Autodesk Inventor part; units mm, degrees
ref_plane "YZ Plane" through (0, 0, 0) normal (1, 0, 0) x (0, 1, 0)
ref_plane "XZ Plane" through (0, 0, 0) normal (0, 1, 0) x (-1, 0, 0)
ref_plane "XY Plane" through (0, 0, 0) normal (0, 0, 1) x (1, 0, 0)
sketch "Sketch1" plane through (0, 0, 0) normal (0, 1, 0) x (-1, 0, 0)
  arc A0 (1.1623, -30.2706) -> (1.1135, 10.0138) centre (15.9463, -10.1104) ccw
  circle A1 centre (15.9463, -10.1104) radius 19
  line L0 (-9.0537, -10.1104) -> (-6.0537, -10.1104)
  line L1 (-6.0537, -10.1104) -> (-6.0537, 49.8896)
  line L2 (-6.0537, 49.8896) -> (-16.0537, 49.8896)
  line L3 (-16.0537, 49.8896) -> (-16.0537, -70.1104)
  line L4 (-16.0537, -70.1104) -> (-6.0537, -70.1104)
  line L5 (-6.0537, -70.1104) -> (-6.0537, -10.1104)
  line L6 (-6.0537, 19.8896) -> (1.1135, 10.0138)
  line L7 (15.9463, -10.1104) -> (15.8318, -10.2667)
  line L8 (1.1623, -30.2706) -> (-6.0537, -40.1104)
  point P0 (0, 0)
  dimension "d0" = 50
  dimension "d1" = 38
  dimension "d2" = 3
  dimension "d4" = 10
  dimension "d5" = 120
  dimension "d11" = 0
extrude "Extrusion1" add sketch "Sketch1" along normal blind 40
sketch "Sketch2" plane through (16.0537, 0, 49.8896) normal (1, 0, 0) x (0, 0, -1)
  line L0 (0, 0) -> (0, 40)
  line L1 (0, 20) -> (120, 20)
  line L2 (120, 0) -> (120, 40)
  circle A0 centre (60, 20) radius 5
  circle A1 centre (20, 20) radius 4
  circle A2 centre (100, 20) radius 4
  point P0 (49.8896, 0)
  dimension "d14" = 10
  dimension "d15" = 8
  dimension "d16" = 8
  dimension "d17" = 20
  dimension "d18" = 20
hole "Hole1" at (16.0537, 20, 29.8896) at (16.0537, 20, -50.1104) direction (-1, 0, 0) diameter 8.376 depth 27.3 tip angle 118
fillet "Fillet1" radius 10 4 edges at (11.0537, 40, 49.8896) (11.0537, 0, 49.8896) (11.0537, 40, -70.1104) (11.0537, 0, -70.1104)
extrude "Extrusion2" cut sketch "Sketch2" against normal blind 100 contours A0 L1 | L1 A0
properties part number "MANCAL_FIXO"
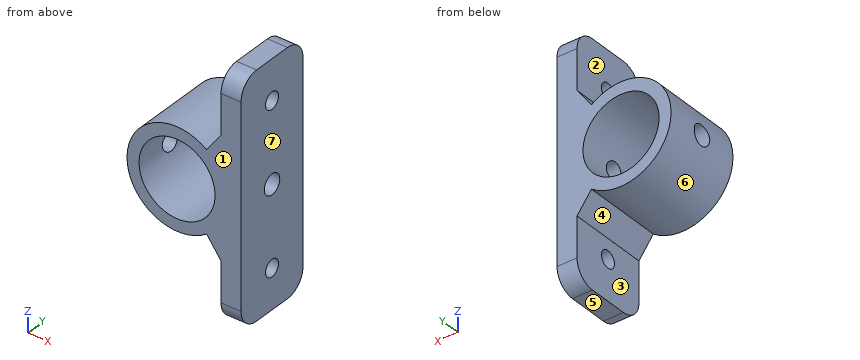
Model file for the job. Use its own axes, mm. Face numbers are marked on the shaded views. A direction names the side the tool comes from. Coordinates: 2 decimals unless noted, no trailing zeros. Write each loop counter-clockwise with the first axis right and the second up, starting at its lowest first coordinate (ties: lowest second). Pieces come first, ordered by that corner, then holes. Notation, with made-up numbers: (53.25, -6) - (109.25, -6) arc R15 cw to (109.25, 14) - close; hole circle Ø2 at (7, 39). An arc over 180 degrees is marked (long way). Use a Markdown table: item, result. Add a question column.
Item 1: Band-saw the part on D-D, the plane x = -32. Write the cut outline in (y, z).
Item 2: Band-saw the part on C-C, the plane y = 21.5. Write the cut outline in (x, z).
Item 3: Drop flat-ended pins along their axis: pin 1 (10 mm diameter, centred on x = -35, y = 14, fed in from +Z); pin 2 (6 mm diameter, centred on y = 20, z = -10.11, fed in from +X); pin 3 (5 mm diameter, centred on y = 27.5, z = 6, fed in from -X); pin 4 (12 mm diameter, centred on x = -13, y = 9.5, fed in from +Z). Give the stop position or say it passes through.
Item 4: Band-saw the part on A-A, the plane x = 8. Write the cut outline in (y, z), and give its area (3 significant figures).
Item 5: Two-plate mould, pull along X, no slides. Class the marked faces 4, 5, 6 and 7: pulls with the +X half, pulls with the -X half, needs draft (parallel to the pull), parting line crosses it, or undercut.
Item 6: Drill centre lines: line 1 along Z through (x, y) = (14, 20); line 2 along Z through (x, y) = (-37.75, 20); line 3 along Z through (x, y) = (-4.5, 10.5). Where is each one in solid material? Low to high.
Item 7: 3-axis set-ups, long thin cutter, end or side, ignore diameter. For the marked faces 1, 2 and 3: which of +Z, -Z, +X, -X, +Y, -Y reach the whole face in a straight line?
Item 8: Band-saw the part on B-B, the plane z = -14. Write the cut outline in (x, y), and give its area (3 significant figures).
A:
| question | item | result |
|---|---|---|
| 1 | outline | (0, -29.27) - (40, -29.27) - (40, -20.27) - (0, -20.27) - close; (0, 0.05) - (40, 0.05) - (40, 9.05) - (0, 9.05) - close |
| 2 | outline | (-40.49, -14.88) arc R25 ccw to (-1.16, -30.27) - (6.05, -40.11) - (6.05, -46.2) - (16.05, -46.2) - (16.05, -14.88) - (2.45, -14.88) arc R19 cw to (-34.34, -14.88) - close; (-40.49, -5.34) - (-34.34, -5.34) arc R19 cw to (2.45, -5.34) - (16.05, -5.34) - (16.05, 25.98) - (6.05, 25.98) - (6.05, 19.89) - (-1.11, 10.01) arc R25 ccw to start; (6.05, -70.11) - (16.05, -70.11) - (16.05, -54.02) - (6.05, -54.02) - close; (6.05, 33.8) - (16.05, 33.8) - (16.05, 49.89) - (6.05, 49.89) - close |
| 3 | pin 1 | stops at z = 10.57 |
| 3 | pin 2 | passes through |
| 3 | pin 3 | stops at x = -36.92 |
| 3 | pin 4 | stops at z = 14.89 |
| 4 | outline | (0, -60.11) arc R10 ccw to (10, -70.11) - (30, -70.11) arc R10 ccw to (40, -60.11) - (40, 39.89) arc R10 ccw to (30, 49.89) - (10, 49.89) arc R10 ccw to (0, 39.89) - close; hole circle Ø10 at (20, -10.11); hole circle Ø8.38 at (20, -50.11); hole circle Ø8.38 at (20, 29.89) |
| 4 | area | 4,530 mm² |
| 5 | face 4 | undercut |
| 5 | face 5 | needs draft |
| 5 | face 6 | undercut |
| 5 | face 7 | pulls with the +X half |
| 6 | line 1 | z = -70.11 to -54.3, -45.92 to -15.11, -5.11 to 25.7, 34.08 to 49.89 |
| 6 | line 2 | z = -22.34 to -15.11, -5.11 to 2.12 |
| 6 | line 3 | z = -32.34 to -25.28, 5.05 to 12.12 |
| 7 | face 1 | +Z, -Z, +X, -X, -Y |
| 7 | face 2 | +Z, -X, +Y, -Y |
| 7 | face 3 | -Z, -X, +Y, -Y |
| 8 | outline | (-40.64, 0) - (-34.54, 0) - (-34.54, 16.86) - (-40.64, 16.86) - close; (-40.64, 23.14) - (-34.54, 23.14) - (-34.54, 40) - (-40.64, 40) - close; (2.65, 0) - (16.05, 0) - (16.05, 16.86) - (2.65, 16.86) - close; (2.65, 23.14) - (16.05, 23.14) - (16.05, 40) - (2.65, 40) - close |
| 8 | area | 657 mm² |
